Geometry: final body of the model. Coordinates: model frame, mm. Face numbers are marked on the shaded views. Coordinates: 2 decimals unless noted, no trailing zeros. Write each loop counter-clockwise with the first axis right and the second up, starting at its lowest first coordinate (ties: lowest second). Pieces come first, ordered by that corner, then holes. Notation, with made-up numbers: (36, 54.25) -> (92, 54.25) arc R22 ccw to (92, 88.25) -> close; hole circle Ø3 at (-9.75, 28.25). An arc over 180 degrees is marked (long way). One line per item, written item: value.
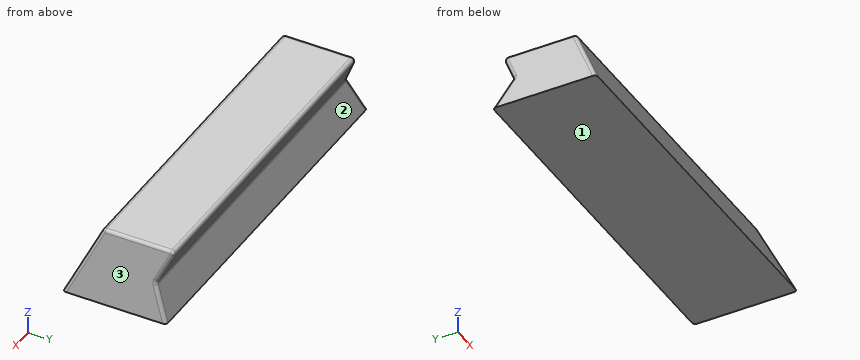
```python
from build123d import *

# Parameters (mm, degrees)
F1_DEPTH = 25
F3_DEPTH = 14.1712295243
F4_R     = 0.5


with BuildPart() as f1:
    # F0 (on Right) → F1 (new body)
    with BuildSketch(Plane.YZ):
        Polygon((4.1702295243, 9.0889595507), (0, 0), (14.1702295243, 0), (12.0851147622, 4.5444797754), (14.1702295243, 9.0889595507), align=None)
    extrude(amount=F1_DEPTH)

    # F2 (on Front) → F3 (cut, through all)
    with BuildSketch(Plane.XZ):
        Polygon((22.5001233071, 9.0889595507), (25.0001233071, 0), (25.0001233071, 9.0889595507), align=None)
    extrude(amount=-F3_DEPTH, mode=Mode.SUBTRACT)

    # F4
    f4_edges = [f1.edges().sort_by_distance(p)[0] for p in [
        (11.250062, 14.17023, 9.08896),
        (11.875062, 12.085115, 4.54448),
        (22.500123, 9.17023, 9.08896),
        (23.125123, 13.127672, 6.81672),
        (23.750062, 2.085218, 4.544704),
        (11.250062, 4.17023, 9.08896),
        (24.375062, 13.127569, 2.272464),
    ]]
    fillet(f4_edges, radius=F4_R)

    # F5: F1 across face


with BuildPart() as f1_1:
    add(f1.part)
    add(f1.part.mirror(Plane(origin=(0, 7.5492536206, 4.2511231401), x_dir=(0, 1, 0), z_dir=(-1, 0, 0))))


solid = f1_1.part
```
(1) Pull-direction query (Z, two-part tool) for the marked faces 1, 2 and 3; classes: released by +Z, released by -Z, zero draft, split by the parting line, or undercut.
Responses:
face 1: released by -Z
face 2: undercut
face 3: released by +Z
(2) First-contact query: pin 1 (2 mm diameter, centred on x = -17.5, z = 7.5, fed in from +Y); pin 2 (3 mm diameter, centred on x = -8.5, z = 8, fed in from -Y); pin 3 (1 mm diameter, centred on x = 16.5, z = 5.5, fed in from -Y). Flat tips, straight axial feed; report the tip coordinate or a pass-through.
Responses:
pin 1: stops at y = 13.88
pin 2: stops at y = 2.98
pin 3: stops at y = 2.29
(3) Line query: line 1 (Z direction, x = 11.5, y = 13.75); line 2 (Z direction, x = -2, y = 12.75); line 3 (X direction, y = 13.5, z = 8). Output: solid intervals per line, ascending. Write a range as [from, to].
Responses:
line 1: z = [0, 0.92], [8.17, 8.94]
line 2: z = [0, 3.1], [5.99, 9.09]
line 3: x = [-22.61, 22.61]
(4) Section B-B (x = 14). Return the cut outline in (y, z).
Responses:
outline: (0, 0) -> (14.17, 0) -> (12.18, 4.34) arc R0.5 cw to (12.18, 4.75) -> (13.85, 8.38) arc R0.5 ccw to (13.39, 9.09) -> (4.49, 9.09) arc R0.5 ccw to (4.04, 8.8) -> close
